Geometry check sheet. Reference: drawing and pictorial views, mm from the part's lowest x, y, z. A direction names the side the tool comes from. Round coordinates to 2 decimals unless told otherwise and drop trailing zeros. Order: outer loops, then holes, each group sorted by start corner. A loop starts at its lowest first (then second) coordinate and runs counter-clockwise, first axis right, second up.
Q1. Set-up check for the marked faces 1, 2 and 3: record each of +Z, -Z, +X, -X, +Y, -Y from which the full face is reachable in a straight line by a thin tool's end or side.
Q2. Cross-section at A-A on z = 1. Record the cut outline in (x, y) (1 decimal).
Q3. Scan lines: probe 1 along Y at (x, z) = (45.5, 3.75); probe 2 along X at (y, z) = (6, 3.05); probe 3 along X at (y, z) = (37, 0.9). Record each from-to range of solid material in increasing order.
Q4. Cross-section at B-B on y = 36. Record the cut outline in (x, z), then the cut area to 3 significant figures.
Q5. Depth check by flat-ended pin: P1, Ø1.9, axis at x = 20, y = 5, coming from the +Z side; P2, Ø2.5, axis at x = 54, z = 3, coming from the -Y side; P3, Ø3, axis at y = 44, z = 0.5, coming from the +X side; P4, Ø2, axis at y = 38.5, z = 3, coming from the -X side. Enter the tip coordinate at first touch or a pass-through.
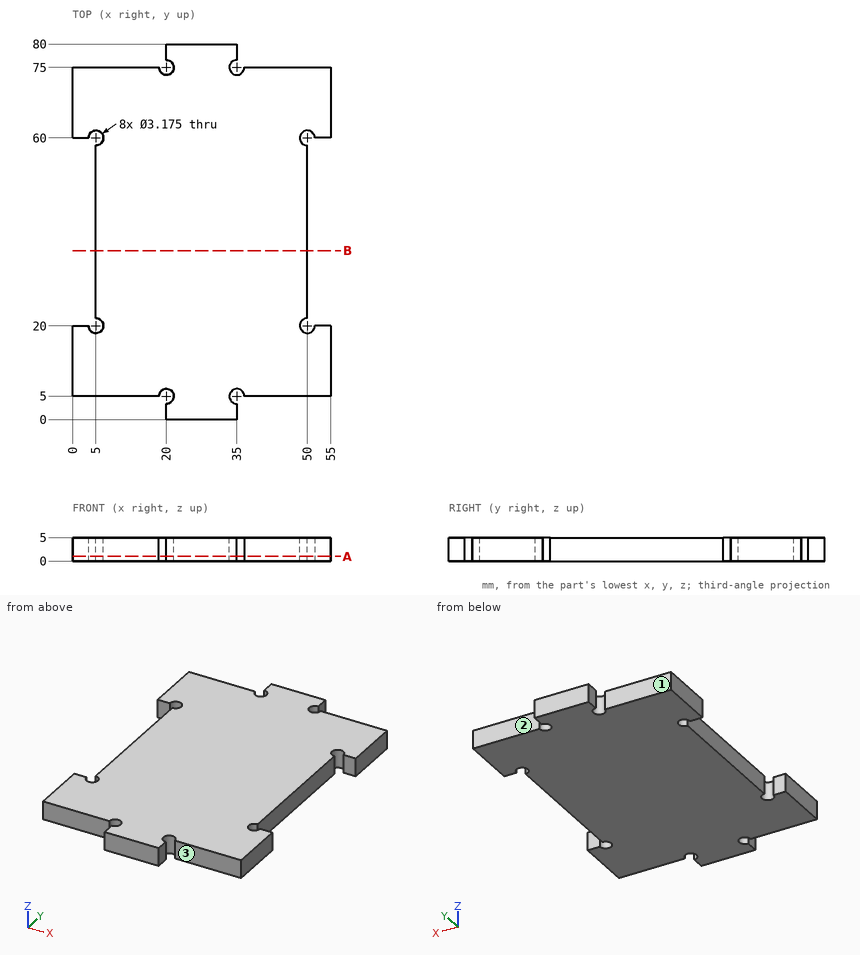
Results found:
1. face 1: +Z, -Z, -X, +Y
1. face 2: +Z, -Z, +X, +Y
1. face 3: +Z, -Z, +X, -Y
2. outline: (0, 5) - (18.4, 5) arc R1.6 cw (long way) to (20, 3.4) - (20, 0) - (35, 0) - (35, 3.4) arc R1.6 cw (long way) to (36.6, 5) - (55, 5) - (55, 20) - (51.6, 20) arc R1.6 cw (long way) to (50, 21.6) - (50, 58.4) arc R1.6 cw (long way) to (51.6, 60) - (55, 60) - (55, 75) - (36.6, 75) arc R1.6 cw (long way) to (35, 76.6) - (35, 80) - (20, 80) - (20, 76.6) arc R1.6 cw (long way) to (18.4, 75) - (0, 75) - (0, 60) - (3.4, 60) arc R1.6 cw (long way) to (5, 58.4) - (5, 21.6) arc R1.6 cw (long way) to (3.4, 20) - (0, 20) - close
3. probe 1: y = 5 to 75
3. probe 2: x = 0 to 18.77, 21.23 to 33.77, 36.23 to 55
3. probe 3: x = 5 to 50
4. outline: (5, 0) - (50, 0) - (50, 5) - (5, 5) - close
4. area: 225 mm2
5. P1: passes through
5. P2: stops at y = 5
5. P3: stops at x = 50
5. P4: stops at x = 5
